The model under review builds one solid part; all positions refer to its coordinate system, in mm. Face numbers are marked on the shaded views. Give positions to 0.01 mm unless a question says otherwise; leave off trailing zeros. Write each loop counter-clockwise with the first axis right and the second up, starting at its lowest first coordinate (ties: lowest second). Pieces come first, ordered by that corner, then holes.
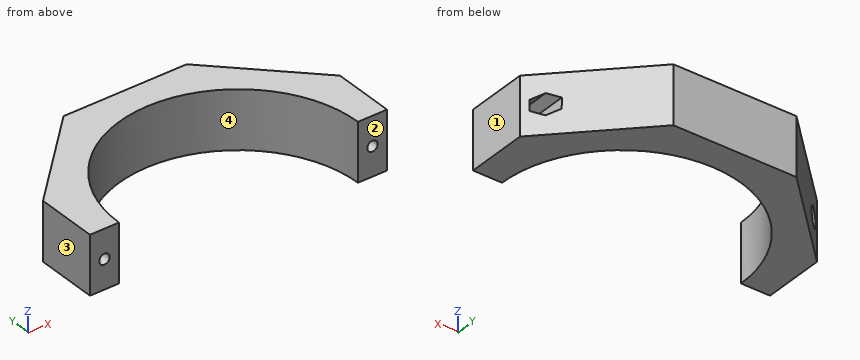
from build123d import *

# Parameters (mm, degrees)
BOSS_EXTRUDE1_DEPTH = 19.05
SKETCH2_R           = 3.429
CUT_EXTRUDE2_DEPTH  = 98.409
SKETCH4_R           = 5.677154031
CUT_EXTRUDE3_DEPTH  = 79.359


with BuildPart() as part:
    # Sketch1 → Boss-Extrude1 (new body, symmetric)
    with BuildSketch(Plane.XY):
        with BuildLine():
            Line((-78.359, 0), (-97.409, 0))
            Line((-97.409, 0), (-97.409, 40.348128897))
            Line((-97.409, 40.348128897), (-40.348128897, 97.409))
            Line((-40.348128897, 97.409), (40.348128897, 97.409))
            Line((40.348128897, 97.409), (97.409, 40.348128897))
            Line((97.409, 40.348128897), (97.409, 0))
            Line((97.409, 0), (78.359, 0))
            ThreePointArc((78.359, 0), (0, 78.359), (-78.359, 0))
        make_face()
    extrude(amount=BOSS_EXTRUDE1_DEPTH, both=True)

    # Sketch2 → Cut-Extrude2 (cut, through all)
    with BuildSketch(Plane.XZ):
        with Locations((87.884, 0)):
            Circle(SKETCH2_R)
        with Locations((-87.884, 0)):
            Circle(SKETCH2_R)
    extrude(amount=-CUT_EXTRUDE2_DEPTH, mode=Mode.SUBTRACT)

    # Sketch4 → Cut-Extrude3 (cut, through all)
    with BuildSketch(Plane(origin=(0, 19.05, 0), x_dir=(-1, 0, 0), z_dir=(0, -1, 0))):
        with Locations((87.884, 0)):
            Circle(SKETCH4_R)
        Polygon((-93.925417492, 3.429), (-93.874309855, -3.517521023), (-87.832892364, -6.946521023), (-81.842582508, -3.429), (-81.893690145, 3.517521023), (-87.935107636, 6.946521023), align=None)
    extrude(amount=-CUT_EXTRUDE3_DEPTH, mode=Mode.SUBTRACT)


solid = part.part
1) To check wall thickness, follow probe 1 along X at (y, z) = (29.5, 0.5); probe 2 along X at (y, z) = (38, 0); probe 3 along X at (y, z) = (25.5, 7.5). State the ranges of each line that lie inside material, in increasing order.
2) The part is to be moulded in two halves that separate along X. For the marked faces 1, 2, 3 and 4, say which applies: +X half, -X half, draft (parallel to the pull), parting line (faces both ways), or undercut.
3) Consider section C-C, the plane z = -11. Give the boundary of the cut face in (x, y).
4) Insertion check: pin 1 (8 mm diameter, centred on x = -87.884, z = 0, fed in from +Y); pin 2 (6 mm diameter, centred on x = 87.884, z = 0, fed in from -Y); pin 3 (4 mm diameter, centred on x = -61, z = 13, fed in from +Y); pin 4 (5 mm diameter, centred on y = 74.5, z = -13, fed in from -X). Each pin has a flat end and moves straight along its axis. Give the tip position at first contact, or say it passes through.
5) Consider section A-A, the plane y = 38. Give the boundary of the cut face in (x, z).
6) Consider section B-B, the plane z = 0. Give the boundary of the cut face in (x, y) (3 decimals).
7) Consider section D-D, the plane x = 0. Give the boundary of the cut face in (y, z), then the cut area to 3 significant figures.
Answer block:
1. probe 1: x = -97.41 to -93.54, -82.23 to -72.59, 72.59 to 81.86, 93.9 to 97.41
1. probe 2: x = -97.41 to -93.56, -82.21 to -68.53, 68.53 to 81.87, 93.9 to 97.41
1. probe 3: x = -97.41 to -74.09, 74.09 to 97.41
2. face 1: +X half
2. face 2: draft
2. face 3: -X half
2. face 4: undercut
3. outline: (-97.41, 0) - (-78.36, 0) arc R78.36 cw to (78.36, 0) - (97.41, 0) - (97.41, 40.35) - (40.35, 97.41) - (-40.35, 97.41) - (-97.41, 40.35) - close
4. pin 1: stops at y = 19.05
4. pin 2: passes through
4. pin 3: stops at y = 78.76
4. pin 4: stops at x = -65.76
5. outline: (-97.41, -19.05) - (-68.53, -19.05) - (-68.53, 19.05) - (-97.41, 19.05) - close; (68.53, -19.05) - (97.41, -19.05) - (97.41, 19.05) - (68.53, 19.05) - close; hole circle Ø11.35 at (-87.88, 0); hole (81.84, 3.43) - (81.89, -3.52) - (87.94, -6.95) - (93.93, -3.43) - (93.87, 3.52) - (87.83, 6.95) - close
6. outline: (-97.409, 0) - (-91.313, 0) - (-91.313, 19.05) - (-93.561, 19.05) - (-93.561, 44.196) - (-97.409, 40.348) - close; (-84.455, 0) - (-78.359, 0) arc R78.359 cw to (78.359, 0) - (84.455, 0) - (84.455, 19.05) - (81.868, 19.05) - (81.868, 55.889) - (40.348, 97.409) - (-40.348, 97.409) - (-82.207, 55.55) - (-82.207, 19.05) - (-84.455, 19.05) - close; (91.313, 0) - (97.409, 0) - (97.409, 40.348) - (93.9, 43.857) - (93.9, 19.05) - (91.313, 19.05) - close
7. outline: (78.36, -19.05) - (97.41, -19.05) - (97.41, 19.05) - (78.36, 19.05) - close
7. area: 726 mm2
